For this review, take the finished solid that the model builds, in its own axes (mm). A direction names the side the tool comes from. Round coordinates to 2 decimals unless told otherwise and drop trailing zeros. Loops run counter-clockwise (first coordinate to the right, second up) from the corner with the lowest first, then second, coordinate; pieces in that order, holes last. Notation, with made-up numbers: (66.25, 60) -> (80.25, 60) arc R25 cw to (80.25, 94) -> close; hole circle Ø8 at (-15.5, 80.5). An arc over 180 degrees is marked (long way). Write each question's results on one line, items separated by ' | '.
```python
from build123d import *

# Parameters (mm, degrees)
F1_DEPTH = 25
F3_DEPTH = 40
F5_DEPTH = 15
F7_DEPTH = 40


with BuildPart() as f1:
    # F0 (on Front) → F1 (new body)
    with BuildSketch(Plane.XZ):
        Polygon((0, 40), (0, 0), (50, 0), align=None)
    extrude(amount=-F1_DEPTH)

    # F2 (on Top) → F3 (join)
    with BuildSketch(Plane.XY):
        Polygon((0, 70), (0, 25), (50, 25), (50, 45), (80, 45), (80, 70), align=None)
    extrude(amount=F3_DEPTH)

    # F4 (on face) → F5 (join)
    with BuildSketch(Plane(origin=(0, 70, 0), x_dir=(-1, 0, 0), z_dir=(0, 1, 0))):
        Polygon((-80, 0), (0, 0), (0, 70), (-30, 70), (-30, 55), (-80, 55), (-80, 40), align=None)
    extrude(amount=F5_DEPTH)

    # F6 (on face) → F7 (cut)
    with BuildSketch(Plane.XY.offset(40)):
        with BuildLine():
            ThreePointArc((27.5, 47.5), (20, 55), (12.5, 47.5))
            ThreePointArc((12.5, 47.5), (20, 40), (27.5, 47.5))
        make_face()
    extrude(amount=-F7_DEPTH, mode=Mode.SUBTRACT)


solid = f1.part
```
1. Consider section B-B (x = 20). State the section outline as (y, z) points, plus the area to 3 significant figures.
Values found:
outline: (0, 0) -> (40, 0) -> (40, 40) -> (25, 40) -> (25, 24) -> (0, 24) -> close; (55, 0) -> (85, 0) -> (85, 70) -> (70, 70) -> (70, 40) -> (55, 40) -> close | area: 2,850 mm2
2. For pin 1 (6 mm diameter, centred on y = 48, z = 45, fed in from +X); pin 2 (13.5 mm diameter, centred on x = 40, y = 53.5, fed in from +Z); pin 3 (15 mm diameter, centred on x = 62, z = 29.5, fed in from -Y); pin 4 (10 mm diameter, centred on x = 31, z = 34.5, fed in from -Y), all flat-tipped, find the tip position at first contact; note any pin that passes through.
Values found:
pin 1: passes through | pin 2: stops at z = 40 | pin 3: stops at y = 45 | pin 4: stops at y = 25
3. Consider section D-D (x = 6). State the section outline as (y, z) points, plus the area to 3 significant figures.
Values found:
outline: (0, 0) -> (85, 0) -> (85, 70) -> (70, 70) -> (70, 40) -> (25, 40) -> (25, 35.2) -> (0, 35.2) -> close | area: 3,730 mm2
4. Tool access review of faces 4 (the face through (36, 25, 29)), 5 (the face through (15, 77, 70)), 6 (the face through (55, 77, 55)), 7 (the face through (65, 45, 20)), 8 (the face through (39, 48, 40)): name each direction out of +Z, -Z, +X, -X, +Y, -Y from which nothing blocks a thin tool from reaching the whole face with its end or side.
Values found:
face 4: +Z, +X, -Y | face 5: +Z, +X, -X, +Y, -Y | face 6: +Z, +X, +Y, -Y | face 7: +Z, -Z, +X, -Y | face 8: +Z, +X, -X, -Y
5. To check wall thickness, follow probe 1 along X at (y, z) = (47, 19); probe 2 along Y at (x, z) = (20, 27); probe 3 along Y at (x, z) = (20, 13). State the ranges of each line that lie inside material, in increasing order.
Values found:
probe 1: x = 0 to 12.52, 27.48 to 80 | probe 2: y = 25 to 40, 55 to 85 | probe 3: y = 0 to 40, 55 to 85
6. Consider section C-C (z = 18). State the section outline as (x, y) points, plus the area to 3 significant figures.
Values found:
outline: (0, 0) -> (27.5, 0) -> (27.5, 25) -> (50, 25) -> (50, 45) -> (80, 45) -> (80, 85) -> (0, 85) -> close; hole circle Ø15 at (20, 47.5) | area: 4,710 mm2
7. Consider section A-A (y = 47.5). State the section outline as (x, z) points, plus the area to 3 significant figures.
Values found:
outline: (0, 0) -> (12.5, 0) -> (12.5, 40) -> (0, 40) -> close; (27.5, 0) -> (80, 0) -> (80, 40) -> (27.5, 40) -> close | area: 2,600 mm2
8. Draft analysis for pull direction X (two halves, no side actions). For faces 1 (the face through (30, 77, 63)), 2 (the face through (0, 51, 27)), 3 (the face through (21.63, 54.82, 20.28)), state which applies: released by +X, released by -X, zero draft, split by the parting line, or undercut.
Values found:
face 1: released by +X | face 2: released by -X | face 3: undercut
